Study the drawing (mm; zero at the part's minimum x, y, z) and answer. A direction names the side the tool comes from. Give positions to 0.01 mm unless a question says otherwise; leave off trailing zeros. Order: outer loops, then holes, each group sorted by start corner. A loop starts at its lowest first (then second) coordinate and runs counter-clockwise, first axis right, second up. Notation, with made-up numbers: (-28, -15.5) -> (15, -15.5) arc R25 cw to (15, 7.5) -> close; hole circle Ø4 at (26, -25.75). An arc over 180 degrees is marked (long way). Use a Markdown table: item, result. Add a question column.
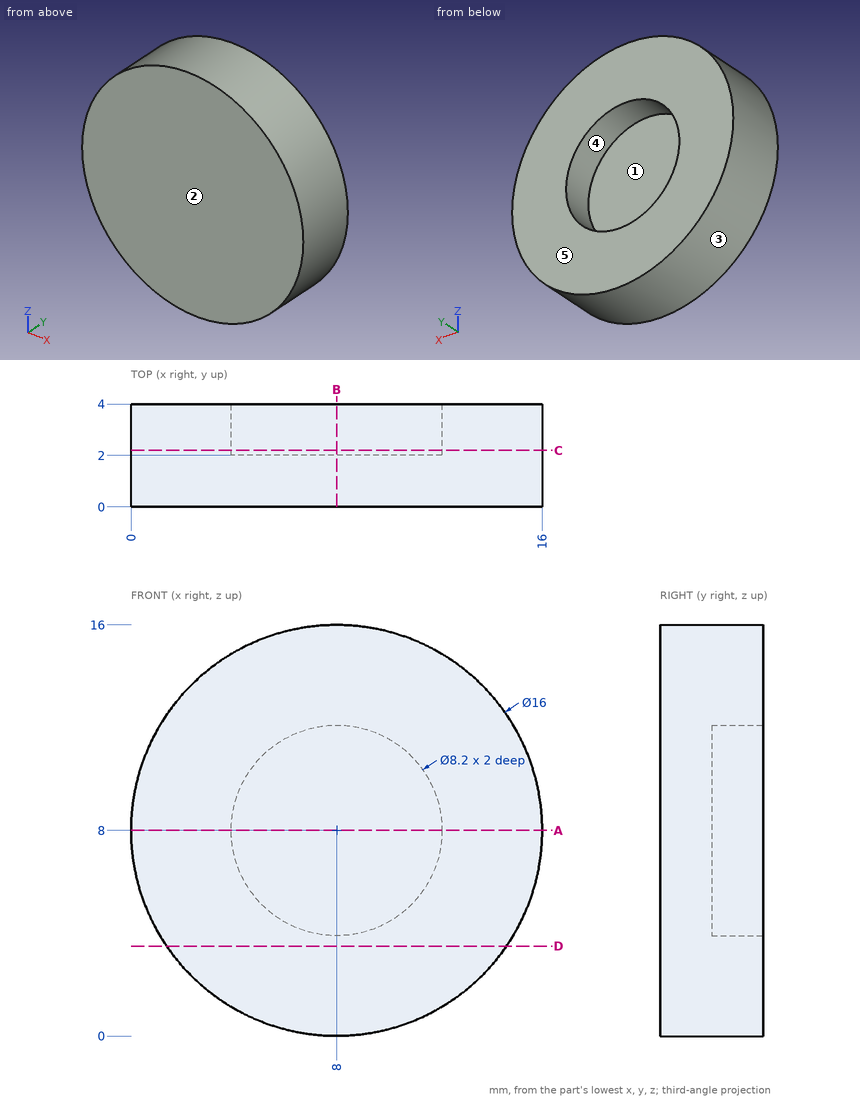
1) The part is cut by section C-C, the plane y = 2.2. Determine the outline of the cut face in (x, z), then the cut area to 3 significant figures.
2) Flat-ended cylindrical pins translate along their axes: pin 1 (2.5 mm diameter, centred on x = 7.5, z = 9.5, fed in from +Y); pin 2 (2 mm diameter, centred on y = 1, z = 12, fed in from -X); pin 3 (2 mm diameter, centred on x = 6, y = 2.5, fed in from -Z). Find the tip coordinate at first contact, or state that the pin passes through.
3) Straight lines are drawn through the part: line 1 (X direction, y = 2.7, z = 8); line 2 (Z direction, x = 11.75, y = 3.55). For each, find the intervals that lie inside material, in ascending order.
4) The part is cut by section D-D, the plane z = 3.5. Determine the outline of the cut face in (x, y), then the cut area to 3 significant figures.
5) Which of the six approach directions +Z, -Z, +X, -X, +Y, -Y give full straight-line access (tool end or side, diameter ignored) to the marked faces 4 and 5?
6) Determine the mould class of the marked faces 1, 2 and 3 for opening direction X: released by +X, released by -X, zero draft, split by the parting line, or undercut.
7) The part is cut by section B-B, the plane x = 8. Determine the outline of the cut face in (y, z).
8) The part is cut by section A-A, the plane z = 8. Determine the outline of the cut face in (x, y), then the cut area to 3 significant figures.
A:
| question | item | result |
|---|---|---|
| 1 | outline | circle Ø16 at (8, 8); hole circle Ø8.2 at (8, 8) |
| 1 | area | 148 mm^2 |
| 2 | pin 1 | y = 2 |
| 2 | pin 2 | x = 0.58 |
| 2 | pin 3 | z = 0.06 |
| 3 | line 1 | 0 to 3.9, 12.1 to 16 |
| 3 | line 2 | 0.93 to 6.34, 9.66 to 15.07 |
| 4 | outline | (1.39, 0) -> (14.61, 0) -> (14.61, 4) -> (1.39, 4) -> close |
| 4 | area | 52.9 mm^2 |
| 5 | face 4 | +Y |
| 5 | face 5 | +Z, -Z, +X, -X, +Y |
| 6 | face 1 | undercut |
| 6 | face 2 | zero draft |
| 6 | face 3 | split by the parting line |
| 7 | outline | (0, 0) -> (4, 0) -> (4, 3.9) -> (2, 3.9) -> (2, 12.1) -> (4, 12.1) -> (4, 16) -> (0, 16) -> close |
| 8 | outline | (0, 0) -> (16, 0) -> (16, 4) -> (12.1, 4) -> (12.1, 2) -> (3.9, 2) -> (3.9, 4) -> (0, 4) -> close |
| 8 | area | 47.6 mm^2 |
